Verification items for the finished model (mm, model axes). A direction names the side the tool comes from. Coordinates: 2 decimals unless noted, no trailing zeros. Order: outer loops, then holes, each group sorted by start corner. A loop starts at its lowest first (then second) coordinate and runs counter-clockwise, first axis right, second up. Notation, with made-up numbers: M 67.25,83 L 85.25,83 A19 cw 85.25,102 Z; hole C -3.5,61.25 d2. An arc over 180 degrees is marked long. Return JSON: item names as keys, results as strings. Group by question number.
Q1. Section check D-D, the plane x = 3. Enter the section's corners in (y, z).
Q2. Thickness scan on probe 1 along Z at (x, y) = (-2.15, 0) (3 decimals); probe 2 along X at (y, z) = (-3.5, 0.75); probe 3 along Y at (x, z) = (8.5, 3.05). Record the ranges inside material, lowest first.
Q3. Section check A-A, the plane y = -6. Enter the section's corners in (x, z), then the cut area to 3 significant figures.
Q4. Section check B-B, the plane x = -1. Enter the section's corners in (y, z) (3 decimals), then the cut area to 3 significant figures.
Q5. Access from +Z, -Z, +X, -X, +Y, -Y to the whole of each face (thin tool, end or side, straight path). Record for faces 4 (the face through (-1.56, -3.45, 2.03)), 5 (the face through (2, 0, -0.5)), 6 (the face through (-2, 0, -0.075)).
Q6. Go/stop test with flat-tipped pins: pin 1 Ø0.6 at (x, y) = (14, 1) entering from +Z; pin 2 Ø2 at (y, z) = (-2, 3.5) entering from +X; pin 3 Ø1.5 at (x, y) = (1, -5) entering from -Z (3 decimals). Record where each tip stops, or that it passes through.
Q7. Section check C-C, the plane y = 0. Enter the section's corners in (x, z) (3 decimals).
Q8. Mould release check, pull along Y, two halves, no side actions. Record for faces 1 (the face through (0.407, -6.499, 1.003)), 2 (the face through (-1.69, 0.2, 3.56)), 3 (the face through (-2, 0, 4.225)): pulls with the +Y half, pulls with the -Y half, needs draft (parallel to the pull), parting line crosses it, or undercut.
from build123d import *

# Parameters (mm, degrees)
F0_W      = 12.8
F0_H      = 7.2
F1_DEPTH  = 4.15
F2_W      = 0.25
F2_H      = 2.5
F2_W_2    = 7.2
F3_DEPTH  = 0.7
F4_R      = 1.5
F5_DEPTH  = 2
F6_SIZE   = 0.25
F7_W      = 1
F7_H      = 3
F8_DEPTH  = 3.35
F9_R      = 1.49999
F10_R     = 0.75
F11_DEPTH = 25
F12_R     = 0.5
F13_DEPTH = 0.5
F14_W     = 0.5
F14_H     = 0.1
F15_DEPTH = 14.45


# Not quite as in the source:
# - a fillet or chamfer is up to 0.001 mm smaller than in the source, because OpenCascade refuses the exact size


with BuildPart() as f1:
    # F0 (on Top) → F1 (new body)
    with BuildSketch(Plane.XY):
        with Locations((6.4, 0)):
            Rectangle(F0_W, F0_H)
    extrude(amount=F1_DEPTH)

    # F2 (on face) → F3 (join)
    with BuildSketch(Plane(origin=(0, 0, 0), x_dir=(0, -1, 0), z_dir=(-1, 0, 0))):
        with BuildLine():
            Line((3.35, 4.74), (-3.35, 4.74))
            ThreePointArc((-3.35, 4.74), (-3.5267766953, 4.6667766953), (-3.6, 4.49))
            Line((-3.6, 4.49), (-3.6, 3.575))
            Line((-3.6, 3.575), (-3.6, 3.325))
            Line((-3.6, 3.325), (3.6, 3.325))
            Line((3.6, 3.325), (3.6, 3.575))
            Line((3.6, 3.575), (3.6, 4.49))
            ThreePointArc((3.6, 4.49), (3.5267766953, 4.6667766953), (3.35, 4.74))
        make_face()
        Polygon((-3.6, 3.325), (-3.6, 3.575), (-3.85, 3.325), align=None)
        Polygon((3.85, 3.325), (3.6, 3.575), (3.6, 3.325), align=None)
        with Locations((-3.725, 2.075)):
            Rectangle(F2_W, F2_H)
        with Locations((3.725, 2.075)):
            Rectangle(F2_W, F2_H)
        with BuildLine():
            Line((3.6, 0.825), (-3.6, 0.825))
            Line((-3.6, 0.825), (-3.6, 0.575))
            Line((-3.6, 0.575), (-3.6, -0.34))
            ThreePointArc((-3.6, -0.34), (-3.5267766953, -0.5167766953), (-3.35, -0.59))
            Line((-3.35, -0.59), (3.35, -0.59))
            ThreePointArc((3.35, -0.59), (3.5267766953, -0.5167766953), (3.6, -0.34))
            Line((3.6, -0.34), (3.6, 0.575))
            Line((3.6, 0.575), (3.6, 0.825))
        make_face()
        Polygon((-3.6, 0.575), (-3.6, 0.825), (-3.85, 0.825), align=None)
        Polygon((3.85, 0.825), (3.6, 0.825), (3.6, 0.575), align=None)
        with Locations((0, 2.075)):
            Rectangle(F2_W_2, F2_H)
    extrude(amount=F3_DEPTH)

    # F4 (on face) → F5 (join)
    with BuildSketch(Plane(origin=(-0.7, 0, 0), x_dir=(0, -1, 0), z_dir=(-1, 0, 0))):
        with BuildLine():
            ThreePointArc((1.3, -0.075), (3.45, 2.075), (1.3, 4.225))
            Line((1.3, 4.225), (-1.3, 4.225))
            ThreePointArc((-1.3, 4.225), (-3.45, 2.075), (-1.3, -0.075))
            Line((-1.3, -0.075), (1.3, -0.075))
        make_face()
        with Locations((0, 2.075)):
            Circle(F4_R, mode=Mode.SUBTRACT)
    extrude(amount=F5_DEPTH)

    # F6
    f6_edges = [f1.edges().sort_by_distance(p)[0] for p in [
        (-2.7, 0, 4.225),
    ]]
    chamfer(f6_edges, length=F6_SIZE)

    # F7 (on face) → F8 (join)
    with BuildSketch(Plane.XZ.offset(3.6)):
        with Locations((0.4, 2.075)):
            Rectangle(F7_W, F7_H)
    extrude(amount=F8_DEPTH)

    # F9 (radius 1.5 in the source; OpenCascade refuses exactly that, so slightly less here)
    f9_edges = [f1.edges().sort_by_distance(p)[0] for p in [
        (0.4, -6.95, 3.575),
        (0.4, -6.95, 0.575),
    ]]
    fillet(f9_edges, radius=F9_R)

    # F10 (on face) → F11 (cut)
    with BuildSketch(Plane(origin=(-0.1, 0, 0), x_dir=(0, -1, 0), z_dir=(-1, 0, 0))):
        with Locations((5.45, 2.075)):
            Circle(F10_R)
    extrude(amount=-F11_DEPTH, mode=Mode.SUBTRACT)

    # F12 (on face) → F13 (join)
    with BuildSketch(Plane(origin=(0, 0, 0), x_dir=(1, 0, 0), z_dir=(0, 0, -1))):
        with Locations((2.3, 0)):
            Circle(F12_R)
        with Locations((7.3, 0)):
            Circle(F12_R)
    extrude(amount=F13_DEPTH)

    # F14 (on face) → F15 (join)
    with BuildSketch(Plane.YZ):
        with Locations((0, 0.05)):
            Rectangle(F14_W, F14_H)
        with Locations((1, 0.05)):
            Rectangle(F14_W, F14_H)
        with Locations((2, 0.05)):
            Rectangle(F14_W, F14_H)
        with Locations((-1, 0.05)):
            Rectangle(F14_W, F14_H)
        with Locations((-2, 0.05)):
            Rectangle(F14_W, F14_H)
    extrude(amount=F15_DEPTH)


solid = f1.part
Numbers:
{
 "1": {"outline": "M -3.6,0 L 3.6,0 L 3.6,4.15 L -3.6,4.15 Z"},
 "2": {"probe 1": "z = -0.075 to 0.575, 3.575 to 4.225", "probe 2": "x = -0.7 to 12.8", "probe 3": "y = -3.6 to 3.6"},
 "3": {"outline": "M -0.1,0.68 L 0.9,0.68 L 0.9,1.57 L -0.1,1.57 Z; M -0.1,2.58 L 0.9,2.58 L 0.9,3.47 L -0.1,3.47 Z", "area": "1.77 mm2"},
 "4": {"outline": "M -1.3,-0.075 L 1.3,-0.075 A2.15 ccw 1.3,4.225 L -1.3,4.225 A2.15 ccw Z; hole C 0,2.075 d3", "area": "18.6 mm2"},
 "5": {"face 4": "-X, -Y", "face 5": "-Z, +X, +Y, -Y", "face 6": "-Z, -X, +Y, -Y"},
 "6": {"pin 1": "stops at z = 0.1", "pin 2": "stops at x = 12.8", "pin 3": "stops at z = 0.575"},
 "7": {"outline": "M -2.7,0.175 L -2.45,-0.075 L -0.7,-0.075 L -0.7,-0.59 L 0,-0.59 L 0,0 L 1.8,0 L 1.8,-0.5 L 2.8,-0.5 L 2.8,0 L 6.8,0 L 6.8,-0.5 L 7.8,-0.5 L 7.8,0 L 14.45,0 L 14.45,0.1 L 12.8,0.1 L 12.8,4.15 L 0,4.15 L 0,4.74 L -0.7,4.74 L -0.7,4.225 L -2.45,4.225 L -2.7,3.975 L -2.7,3.575 L -0.7,3.575 L -0.7,0.575 L -2.7,0.575 Z"},
 "8": {"face 1": "pulls with the -Y half", "face 2": "undercut", "face 3": "needs draft"}
}
